The model under review builds one solid part; all positions refer to its coordinate system, in mm. A direction names the side the tool comes from. Coordinates: 2 decimals unless noted, no trailing zeros. Loops run counter-clockwise (first coordinate to the right, second up) from the corner with the lowest first, then second, coordinate; pieces in that order, holes last. Notation, with made-up numbers: M 73,19.5 L 96,19.5 A34 cw 96,50.5 Z; hole C 36,76.25 d11. An arc over 180 degrees is marked long. Return JSON: item names as keys, results as strings.
Autodesk Fusion 360 part; units mm, degrees
sketch "Esquisse1" plane through (0, 0, 0) normal (0, 0, 1) x (1, 0, 0)
  line L0 (0, 0) -> (50, 0)
  line L1 (50, 0) -> (50, 50)
  line L2 (50, 50) -> (0, 50)
  line L3 (0, 50) -> (0, 0)
  dimension "d1" = 50
  dimension "d2" = 50
extrude "Extrusion1" add sketch "Esquisse1" along normal blind 2.7
sketch "Esquisse2" plane through (0, 0, 0) normal (0, 1, 0) x (1, 0, 0)
  line L0 (0, -50) -> (50, -50)
  line L1 (50, -50) -> (50, 0)
  line L2 (50, 0) -> (0, 0)
  line L3 (0, 0) -> (0, -50)
extrude "Extrusion2" add sketch "Esquisse2" against normal blind 2.7
sketch "Esquisse3" plane through (0, 0, 2.7) normal (0, 0, 1) x (-1, 0, 0)
  line L0 (0, -50) -> (0, 0)
  line L1 (0, 0) -> (-50, 0)
  line L2 (-50, 0) -> (-50, -50)
  line L3 (-50, -50) -> (0, -50)
  circle A0 centre (-25, -25) radius 11
  dimension "d7" = 22
extrude "Extrusion3" cut sketch "Esquisse3" against normal blind 10 contours A0
sketch "Esquisse4" plane through (0, 0, 2.7) normal (0, 0, 1) x (-1, 0, 0)
  circle A0 centre (-25, -25) radius 11
  line L0 (0, -50) -> (0, 0)
  line L1 (0, 0) -> (-50, 0)
  line L2 (-50, 0) -> (-50, -50)
  line L3 (-50, -50) -> (0, -50)
  circle A1 centre (-9.5, -40.5) radius 2
  dimension "d10" = 4
  dimension "d11" = 15.5
  dimension "d12" = 15.5
extrude "Extrusion4" cut sketch "Esquisse4" against normal blind 10 contours A1
pattern_linear "Réseau R1" count 2 spacing 31 along (1, 0, 0) count 2 spacing 31 along (0, -1, 0) of "Extrusion4"
sketch "Esquisse5" plane through (0, 0, 0) normal (0, 1, 0) x (-1, 0, 0)
  line L0 (-50, 2.7) -> (0, 2.7)
  line L1 (0, 2.7) -> (0, 50)
  line L2 (0, 50) -> (-50, 50)
  line L3 (-50, 50) -> (-50, 2.7)
  line L4 (-42.65, 9.1521) -> (-42.65, 43.1521)
  arc A0 (-38.35, 43.1521) -> (-42.65, 43.1521) centre (-40.5, 43.1521) ccw
  line L5 (-38.35, 43.1521) -> (-38.35, 9.1521)
  arc A1 (-42.65, 9.1521) -> (-38.35, 9.1521) centre (-40.5, 9.1521) ccw
  dimension "d19" = 4.3
  dimension "d20" = 34
  dimension "d22" = 9.5
extrude "Extrusion5" cut sketch "Esquisse5" against normal blind 6 contours L4 A0 L5 A1
pattern_linear "Réseau R2" count 2 spacing 31 along (-1, 0, 0) of "Extrusion5"
chamfer "Chanfrein1" distance 4 angle 45 4 edges at (50, -1.35, 50) (0, -1.35, 50) (50, 50, 1.35) (0, 50, 1.35)
equation "d11 = ( 31 / 2 ) * 1 mm"
equation "d12 = ( 31 / 2 ) * 1 mm"
1. Add section B-B on y = 40.5. Give the boundary of the cut face in (x, z).
Check values:
{"outline": "M 0,0 L 7.5,0 L 7.5,2.7 L 0,2.7 Z; M 11.5,0 L 38.5,0 L 38.5,2.7 L 11.5,2.7 Z; M 42.5,0 L 50,0 L 50,2.7 L 42.5,2.7 Z"}
2. The part is to be moulded in two halves that separate along X. For faces 1 (the face through (25, -2.7, 25)), 2 (the face through (9.45, -1.33, 45.3)), 3 (the face through (2, -1, 48)), say which applies: released by +X, released by -X, zero draft, split by the parting line, or undercut.
Check values:
{"face 1": "zero draft", "face 2": "undercut", "face 3": "released by -X"}
3. Add section A-A on x = 40.5. Give the boundary of the cut face in (y, z), plus the area to 3 significant figures.
Check values:
{"outline": "M -2.7,0 L 7.5,0 L 7.5,2.7 L 0,2.7 L 0,7 L -2.7,7 Z; M -2.7,45.3 L 0,45.3 L 0,50 L -2.7,50 Z; M 11.5,0 L 38.5,0 L 38.5,2.7 L 11.5,2.7 Z; M 42.5,0 L 50,0 L 50,2.7 L 42.5,2.7 Z", "area": "145 mm²"}
4. Insertion check: pin 1 Ø23.5 at (x, z) = (35, 16.5) entering from +Y; pin 2 Ø5 at (x, y) = (9.5, 9.5) entering from +Z. Each pin has a flat end and moves straight along its axis. Give the tip position at first contact, or say it passes through.
Check values:
{"pin 1": "y = 0", "pin 2": "z = 2.7"}
5. Add section D-D on y = 25. Give the boundary of the cut face in (x, z), plus the area to 3 significant figures.
Check values:
{"outline": "M 0,0 L 14,0 L 14,2.7 L 0,2.7 Z; M 36,0 L 50,0 L 50,2.7 L 36,2.7 Z", "area": "75.6 mm²"}
6. Add section C-C on x = 25. Give the boundary of the cut face in (y, z).
Check values:
{"outline": "M -2.7,0 L 14,0 L 14,2.7 L 0,2.7 L 0,50 L -2.7,50 Z; M 36,0 L 50,0 L 50,2.7 L 36,2.7 Z"}
7. Machinability: for faces 4 (the face through (48, -1, 48)), 5 (the face through (25, 0, 26)), 6 (the face through (9.547, -1.331, 7.003)), which of the approach directions +Z, -Z, +X, -X, +Y, -Y give a long, thin tool a straight path to every point of the face, cutting with its end or side? Answer none if there is none.
Check values:
{"face 4": "+Z, +X, +Y, -Y", "face 5": "+Z, +X, -X, +Y", "face 6": "+Y, -Y"}
8. To check wall thickness, follow line 1 (X direction, y = 9.5, z = 1.1); line 2 (Y direction, x = 40.5, z = 0.85); line 3 (X direction, y = 25, z = 2.1). State the ranges of each line that lie inside material, in increasing order.
Check values:
{"line 1": "0 to 7.5, 11.5 to 38.5, 42.5 to 50", "line 2": "-2.7 to 7.5, 11.5 to 38.5, 42.5 to 50", "line 3": "0 to 14, 36 to 50"}
